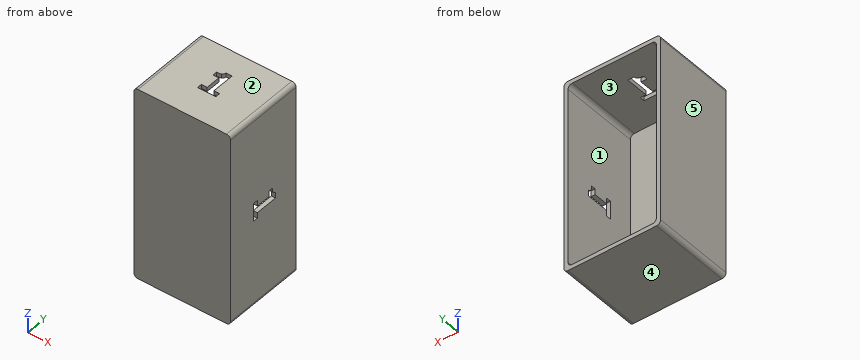
Autodesk Inventor part; units mm, degrees
ref_plane "YZ Plane" through (0, 0, 0) normal (1, 0, 0) x (0, 1, 0)
ref_plane "XZ Plane" through (0, 0, 0) normal (0, 1, 0) x (-1, 0, 0)
ref_plane "XY Plane" through (0, 0, 0) normal (0, 0, 1) x (1, 0, 0)
sketch "Эскиз1" plane through (0, 0, 0) normal (0, 1, 0) x (-1, 0, 0)
  line L0 (0, 0) -> (-70, 0)
  line L1 (-70, 0) -> (-70, -140)
  line L2 (-70, -140) -> (0, -140)
  line L3 (0, -140) -> (0, 0)
  dimension "d0" = 70
  dimension "d1" = 140
extrude "Выдавливание1" add sketch "Эскиз1" along normal blind 60
shell "Оболочка1" thickness 3 removed faces 1 at (46.6667, 60, -93.3333)
sketch "Эскиз2" plane through (70, 0, 0) normal (1, 0, 0) x (0, 0, -1)
  line L0 (0, 60) -> (140, 60)
  line L1 (60.8364, 41.1842) -> (78.3566, 41.1842) construction
  line L2 (78.3566, 41.1842) -> (78.3566, 21.1356) construction
  line L3 (78.3566, 21.1356) -> (60.8364, 21.1356) construction
  line L4 (60.8364, 21.1356) -> (60.8364, 41.1842) construction
  line L5 (76.6711, 21.1356) -> (63.462, 21.1356)
  line L6 (63.462, 21.1356) -> (63.462, 24.6202)
  line L7 (63.462, 24.6202) -> (67.6759, 24.6202)
  line L8 (67.6759, 24.6202) -> (67.6759, 35.2037)
  line L9 (67.6759, 35.2037) -> (63.462, 35.2037)
  line L10 (63.462, 35.2037) -> (63.462, 38.4614)
  spline S0 degree 2 poles (63.462, 38.4614) (64.3858, 38.4614) (66.2172, 38.7045) (66.7683, 38.9638) knots 0 0 0 1 2 2 2
  spline S1 degree 2 poles (66.7683, 38.9638) (67.4004, 39.288) (68.1135, 40.3739) (68.1784, 41.1842) knots 0 0 0 1 2 2 2
  line L11 (68.1784, 41.1842) -> (72.5544, 41.1842)
  line L12 (72.5544, 41.1842) -> (72.5544, 24.6202)
  line L13 (72.5544, 24.6202) -> (76.6711, 24.6202)
  line L14 (76.6711, 24.6202) -> (76.6711, 21.1356)
  point P0 (0, 0)
  point P1 (70, 30.2829)
extrude "Выдавливание2" cut sketch "Эскиз2" against normal blind 12
sketch "Эскиз3" plane through (0, 0, 0) normal (0, 0, 1) x (1, 0, 0)
  line L0 (0, 60) -> (70, 60)
  line L1 (25.7932, 42.4372) -> (43.3135, 42.4372) construction
  line L2 (43.3135, 42.4372) -> (43.3135, 22.3886) construction
  line L3 (43.3135, 22.3886) -> (25.7932, 22.3886) construction
  line L4 (25.7932, 22.3886) -> (25.7932, 42.4372) construction
  line L5 (41.6279, 22.3886) -> (28.4189, 22.3886)
  line L6 (28.4189, 22.3886) -> (28.4189, 25.8732)
  line L7 (28.4189, 25.8732) -> (32.6328, 25.8732)
  line L8 (32.6328, 25.8732) -> (32.6328, 36.4566)
  line L9 (32.6328, 36.4566) -> (28.4189, 36.4566)
  line L10 (28.4189, 36.4566) -> (28.4189, 39.7143)
  spline S0 degree 2 poles (28.4189, 39.7143) (29.3427, 39.7143) (31.1741, 39.9575) (31.7252, 40.2168) knots 0 0 0 1 2 2 2
  spline S1 degree 2 poles (31.7252, 40.2168) (32.3573, 40.5409) (33.0704, 41.6268) (33.1352, 42.4372) knots 0 0 0 1 2 2 2
  line L11 (33.1352, 42.4372) -> (37.5112, 42.4372)
  line L12 (37.5112, 42.4372) -> (37.5112, 25.8732)
  line L13 (37.5112, 25.8732) -> (41.6279, 25.8732)
  line L14 (41.6279, 25.8732) -> (41.6279, 22.3886)
  point P0 (0, 0)
  point P1 (35, 31.2439)
extrude "Выдавливание3" cut sketch "Эскиз3" against normal blind 12
fillet "Сопряжение1" radius 3 4 edges at (3, 31.5, -3) (67, 31.5, -3) (3, 31.5, -137) (67, 31.5, -137)
fillet "Сопряжение2" radius 3 4 edges at (0, 30, -140) (0, 30, 0) (70, 30, -140) (70, 30, 0)
properties part number "Контейнер 1"
Design review of the part built by this model. Coordinates are the model's own, in mm. Face numbers are marked on the shaded views. A direction names the side the tool comes from. Coordinates: 2 decimals unless noted, no trailing zeros. Order: outer loops, then holes, each group sorted by start corner. A loop starts at its lowest first (then second) coordinate and runs counter-clockwise, first axis right, second up. Notation, with made-up numbers: M 42,69.25 L 91,69.25 A14 cw 91,74.25 Z; hole C 9.5,29.5 d7. An arc over 180 degrees is marked long. Answer as a JSON object with one key per item and string values. Group by question number.
1) Tool access review of the marked faces 1 and 2: name each direction out of +Z, -Z, +X, -X, +Y, -Y from which nothing blocks a thin tool from reaching the whole face with its end or side.
2) Add section C-C, the plane y = 27.5. Write out the cut boundary in (x, z), then the cut area to 3 significant figures.
3) Add section D-D, the plane z = -101. Write out the cut boundary in (x, y), then the cut area to 3 significant figures.
4) Add section B-B, the plane y = 46. Write out the cut boundary in (x, z).
5) For pin 1 (0.9 mm diameter, centred on x = 68.5, y = 29.5, fed in from +Z); pin 2 (5 mm diameter, centred on x = 32.5, z = -71, fed in from +Y); pin 3 (0.9 mm diameter, centred on x = 68, y = 22.5, fed in from +Z), all flat-tipped, find the tip position at first contact; note any pin that passes through.
6) Add section A-A, the plane x = 36. Write out the cut boundary in (y, z), then the cut area to 3 significant figures.
7) Mouldability with a two-part tool opening along X and no side actions: class the marked faces 3, 4 and 5 as pulls with the +X half, pulls with the -X half, needs draft (parallel to the pull), parting line crosses it, or undercut.
8) Wall thickness on L1, parallel to Z at x = 14, y = 46; L2, parallel to X at y = 55, z = -50.5; L3, parallel to Y at x = 32.5, z = -115: over which ranges is each line inside the solid? List them lowest first.
Computed values:
{
 "1": {"face 1": "+Y", "face 2": "+Z, +X, -X, +Y, -Y"},
 "2": {"outline": "M 0,-137 A3 ccw 3,-140 L 67,-140 A3 ccw 70,-137 L 70,-72.55 L 67,-72.55 L 67,-134 A3 cw 64,-137 L 6,-137 A3 cw 3,-134 L 3,-6 A3 cw 6,-3 L 32.63,-3 L 32.63,0 L 3,0 A3 ccw 0,-3 Z; M 37.51,-3 L 64,-3 A3 cw 67,-6 L 67,-67.68 L 70,-67.68 L 70,-3 A3 ccw 67,0 L 37.51,0 Z", "area": "1,190 mm^2"},
 "3": {"outline": "M 0,0 L 70,0 L 70,60 L 67,60 L 67,3 L 3,3 L 3,60 L 0,60 Z", "area": "552 mm^2"},
 "4": {"outline": "M 0,-137 A3 ccw 3,-140 L 67,-140 A3 ccw 70,-137 L 70,-3 A3 ccw 67,0 L 3,0 A3 ccw 0,-3 Z; hole M 3,-134 A3 ccw 6,-137 L 64,-137 A3 ccw 67,-134 L 67,-6 A3 ccw 64,-3 L 6,-3 A3 ccw 3,-6 Z"},
 "5": {"pin 1": "stops at z = -0.19", "pin 2": "stops at y = 3", "pin 3": "stops at z = -0.05"},
 "6": {"outline": "M 0,-140 L 60,-140 L 60,-137 L 3,-137 L 3,-3 L 22.39,-3 L 22.39,0 L 0,0 Z; M 42.44,-3 L 60,-3 L 60,0 L 42.44,0 Z", "area": "702 mm^2"},
 "7": {"face 3": "undercut", "face 4": "needs draft", "face 5": "pulls with the -X half"},
 "8": {"L1": "z = -140 to -137, -3 to 0", "L2": "x = 0 to 3, 67 to 70", "L3": "y = 0 to 3"}
}
